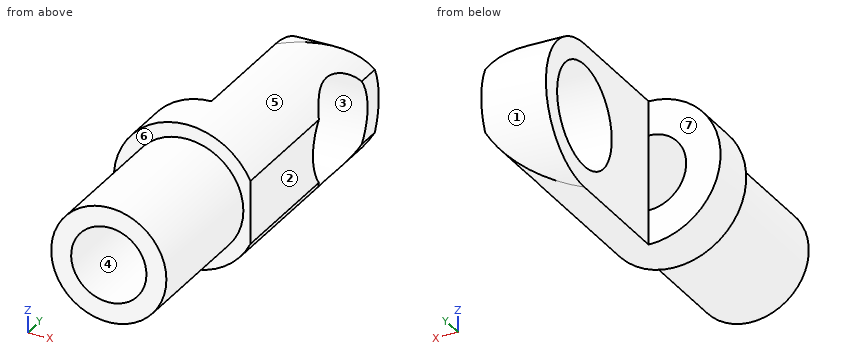
Autodesk Inventor part; units mm, degrees
ref_plane "YZ Plane" through (0, 0, 0) normal (1, 0, 0) x (0, 1, 0)
ref_plane "XZ Plane" through (0, 0, 0) normal (0, 1, 0) x (-1, 0, 0)
ref_plane "XY Plane" through (0, 0, 0) normal (0, 0, 1) x (1, 0, 0)
sketch "Sketch1" plane through (0, 0, 0) normal (0, 1, 0) x (-1, 0, 0)
  circle A0 centre (0, 0) radius 4.7625
  dimension "d0" = 9.525
extrude "Extrusion1" add sketch "Sketch1" along normal blind 12.7
sketch "Sketch2" plane through (0, 0, 0) normal (0, -1, 0) x (1, 0, 0)
  circle A0 centre (0, 0) radius 2.539
hole "Hole1" at (0, 0, 0) direction (0, 1, 0) diameter 4.9784 depth 19.05 tip angle 118
sketch "Sketch3" plane through (0, 12.7, 0) normal (0, 1, 0) x (1, 0, 0)
  circle A0 centre (0, 0) radius 4.7625
  circle A1 centre (0, 0) radius 4.7625
  line L0 (0, -4.7625) -> (0, 4.7625)
  dimension "d10" = 9.525
extrude "Extrusion2" add sketch "Sketch3" along normal blind 12.7 contours A0 L0 picked at (1.6786, -1.3984)
sketch "Sketch4" plane through (0, 12.7, -2.4892) normal (-1, 0, 0) x (0, 0, 1)
  line L0 (-2.2733, 0) -> (-2.2733, 12.7)
  line L1 (7.2517, 0) -> (7.2517, 12.7)
  line L2 (-2.2733, 0) -> (7.2517, 0)
  line L3 (7.2517, 0) -> (7.2517, 12.7)
  line L4 (7.2517, 12.7) -> (-2.2733, 12.7)
  line L5 (-2.2733, 12.7) -> (-2.2733, 0)
  arc A0 (7.2517, 7.9375) -> (-2.2733, 7.9375) centre (2.4892, 7.9375) ccw
  line L6 (7.2517, 12.7) -> (-2.2733, 12.7)
  line L7 (-2.2733, 7.9375) -> (-2.2733, 12.7)
  line L8 (-2.2733, 12.7) -> (7.2517, 12.7)
  line L9 (7.2517, 12.7) -> (7.2517, 7.9375)
  point P0 (2.4892, -12.7)
extrude "Extrusion3" cut sketch "Sketch4" against normal blind 12.7 contours L0 L4 A0 | L4 L1 A0
sketch "Sketch5" plane through (0, 12.7, -2.4892) normal (-1, 0, 0) x (0, 0, 1)
  arc A0 (7.2517, 7.9375) -> (-2.2733, 7.9375) centre (2.4892, 7.9375) ccw
  circle A1 centre (2.4892, 7.9375) radius 2.2013
  point P0 (2.4892, -12.7)
hole "Hole2" at (0, 20.6375, 0) direction (1, 0, 0) diameter 6.7564 depth 19.05 tip angle 118
sketch "Sketch6" plane through (0, 0, 0) normal (0, -1, 0) x (1, 0, 0)
  line L0 (0, 0) -> (4.7909, 0)
  line L1 (5.3024, 5.1468) -> (4.2794, 5.1468)
  line L2 (4.2794, 5.1468) -> (4.2794, -5.1468)
  line L3 (4.2794, -5.1468) -> (5.3024, -5.1468)
  line L4 (5.3024, -5.1468) -> (5.3024, 5.1468)
  line L5 (5.3024, 5.1468) -> (4.2794, -5.1468) construction
  line L6 (4.2794, 5.1468) -> (5.3024, -5.1468) construction
extrude "Extrusion4" cut sketch "Sketch6" against normal blind 25.4
sketch "Sketch7" plane through (0, 0, 0) normal (0, -1, 0) x (1, 0, 0)
  circle A0 centre (0, 0) radius 4.7625
  circle A1 centre (0, 0) radius 3.81
  dimension "d24" = 9.525
  dimension "d25" = 7.62
extrude "Extrusion5" cut sketch "Sketch7" against normal blind 9.525
properties part number "feet type 3 part 2" material "Stainless Steel"
Work out the finished part from the listing and answer in its coordinate system (mm). Face numbers are marked on the shaded views. A direction names the side the tool comes from. Coordinates: 2 decimals unless noted, no trailing zeros. Write each loop counter-clockwise with the first axis right and the second up, starting at its lowest first coordinate (ties: lowest second). Pieces come first, ordered by that corner, then holes. Notation, with made-up numbers: M 63.5,24 L 108.5,24 A28 cw 108.5,45 Z; hole C -1.5,-34 d5. An arc over 180 degrees is marked long. Answer as CSV lines item,"result". Start each with the question number.
Item 1: Section C-C on z = 3 is taken. Write down the section's boundary in (x, y) (3 decimals), and give its area (3 significant figures).
Item 2: Flat-ended cylindrical pins translate along their axes: P1, Ø1.5, axis at y = 21, z = -2.5, coming from the -X side; P2, Ø1, axis at x = 0.5, y = 5, coming from the +Z side; P3, Ø4, axis at x = 0, z = 0, coming from the -Y side; P4, Ø5, axis at y = 11, z = -3.5, coming from the -X side. Find the tip coordinate at first contact, or state that the pin passes through.
Item 3: A tool of negligible diameter and unlimited length cuts with its end or side. For the marked faces 5, 6 and 7, from which of +Z, -Z, +X, -X, +Y, -Y can it reach the whole face along a straight path? Write none if from no direction.
Item 4: Section D-D on x = 1.25 is taken. Write down the section's boundary in (y, z) (1 decimal).
Item 5: Consider L1, parallel to Y at x = 2.45, z = 0; L2, parallel to Z at x = 0, y = 6.75; L3, parallel to Z at x = 1, y = 10. Determine where each line is inside the solid, lowest interval first.
Item 6: Determine the mould class of the marked faces 1, 2, 3 and 4 for opening direction Z: released by +Z, released by -Z, zero draft, split by the parting line, or undercut.
Item 7: Section B-B on y = 19.5 is taken. Write down the section's boundary in (x, z) (1 decimal).
Item 8: Section A-A on z = 0 is taken. Write down the section's boundary in (x, y) (1 decimal), and give its area (3 significant figures).
Checks:
1,outline,"M -3.699,9.525 L -2.349,9.525 L -2.349,0 L 2.349,0 L 2.349,9.525 L 3.699,9.525 L 3.699,19.084 L 0,19.084 L 0,12.7 L -3.699,12.7 Z; M 0,22.191 L 3.699,22.191 L 3.699,24.336 L 0,24.336 Z"
1,area,"99.8 mm²"
2,P1,"passes through"
2,P2,"stops at z = 3.81"
2,P3,"stops at y = 12.7"
2,P4,"stops at x = -4.66"
3,face 5,"+Y, -Y"
3,face 6,"-Y"
3,face 7,"+Z, -Z, -X, +Y"
4,outline,"M 0,-3.6 L 9.5,-3.6 L 9.5,-4.6 L 21.9,-4.6 A4.8 ccw 21.9,4.6 L 9.5,4.6 L 9.5,3.6 L 0,3.6 L 0,2.2 L 12.7,2.2 L 12.7,-2.2 L 0,-2.2 Z; hole C 20.6,0 d6.8"
5,L1,"y = 12.7 to 17.26, 24.02 to 25.4"
5,L2,"z = -3.81 to -2.49, 2.49 to 3.81"
5,L3,"z = -4.66 to -2.28, 2.28 to 4.66"
6,face 1,"split by the parting line"
6,face 2,"zero draft"
6,face 3,"undercut"
6,face 4,"undercut"
7,outline,"M 0,-4.8 A4.8 ccw 3.5,-3.2 L 0,-3.2 Z; M 0,3.2 L 3.5,3.2 A4.8 ccw 0,4.8 Z"
8,outline,"M -4.8,9.5 L -3.8,9.5 L -3.8,0 L -2.5,0 L -2.5,12.7 L -4.8,12.7 Z; M 0,12.7 L 2.5,12.7 L 2.5,0 L 3.8,0 L 3.8,9.5 L 4.3,9.5 L 4.3,17.3 L 0,17.3 Z; M 0,24 L 4.3,24 L 4.3,25.4 L 0,25.4 Z"
8,area,"63.5 mm²"
